Autodesk Inventor part; units mm, degrees
ref_plane "YZ Plane" through (0, 0, 0) normal (1, 0, 0) x (0, 1, 0)
ref_plane "XZ Plane" through (0, 0, 0) normal (0, 1, 0) x (-1, 0, 0)
ref_plane "XY Plane" through (0, 0, 0) normal (0, 0, 1) x (1, 0, 0)
sketch "Эскиз1" plane through (0, 0, 0) normal (0, 0, 1) x (1, 0, 0)
  line L0 (0, 0) -> (35, 0)
  line L1 (35, 0) -> (35, 50)
  line L2 (35, 50) -> (0, 50)
  line L3 (0, 50) -> (0, 0)
  dimension "d0" = 35
  dimension "d1" = 50
extrude "Выдавливание1" add sketch "Эскиз1" along normal blind 1.8
sketch "Эскиз2" plane through (0, 0, 1.8) normal (0, 0, 1) x (1, 0, 0)
  line L0 (0, 0) -> (35, 0)
  line L1 (35, 0) -> (35, 1.8)
  line L2 (35, 1.8) -> (0, 1.8)
  line L3 (0, 1.8) -> (0, 0)
  dimension "d5" = 35
  dimension "d6" = 1.8
extrude "Выдавливание2" add sketch "Эскиз2" along normal blind 48.2
fillet "Сопряжение1" radius 2 2 edges at (17.5, 1.8, 1.8) (17.5, 0, 0)
chamfer "Фаска1" distance 5.175 angle 45 4 edges at (0, 50, 0.9) (0, 0.9, 50) (35, 0.9, 50) (35, 50, 0.9)
sketch "Эскиз3" plane through (0, 0, 1.8) normal (0, 0, 1) x (1, 0, 0)
  line L0 (29.825, 50) -> (5.175, 50)
  line L1 (17.5, 50) -> (17.5, 1.8)
  line L2 (0, 1.8) -> (35, 1.8)
  line L3 (29.825, 50) -> (5.175, 50)
  circle A0 centre (17.5, 39.6875) radius 5
  circle A1 centre (7.9375, 44.6875) radius 2
  circle A2 centre (26.9875, 44.6875) radius 2
  circle A3 centre (5.175, 33.3375) radius 2
  circle A4 centre (29.825, 33.3375) radius 2
  circle A5 centre (7.9375, 20.6375) radius 2
  circle A6 centre (26.9875, 20.6375) radius 2
  point P0 (0, 0)
  dimension "d14" = 10
  dimension "d15" = 4
  dimension "d16" = 4
  dimension "d17" = 4
  dimension "d18" = 4
  dimension "d19" = 4
  dimension "d20" = 4
extrude "Выдавливание3" cut sketch "Эскиз3" against normal blind 48.2
sketch "Эскиз4" plane through (0, 1.8, 3.8) normal (0, 1, 0) x (1, 0, 0)
  line L0 (5.175, -46.2) -> (29.825, -46.2)
  line L1 (5.175, -46.2) -> (29.825, -46.2)
  circle A0 centre (17.5, -35.8875) radius 5
  circle A1 centre (27.0625, -40.8875) radius 2
  circle A2 centre (8.0125, -40.8875) radius 2
  circle A3 centre (29.825, -29.5375) radius 2
  circle A4 centre (5.175, -29.5375) radius 2
  circle A5 centre (27.0625, -16.8375) radius 2
  circle A6 centre (8.0125, -16.8375) radius 2
  line L2 (29.825, -46.2) -> (5.175, -46.2)
  point P0 (0, 3.8)
  point P1 (17.5, -46.2)
  dimension "d23" = 10
  dimension "d24" = 4
  dimension "d25" = 4
  dimension "d26" = 4
  dimension "d27" = 4
  dimension "d28" = 4
  dimension "d29" = 4
extrude "Выдавливание4" cut sketch "Эскиз4" against normal blind 48.2
properties part number "угол для катушки"
Model file for the job. Use its own axes, mm. A direction names the side the tool comes from. Coordinates: 2 decimals unless noted, no trailing zeros. Write each loop counter-clockwise with the first axis right and the second up, starting at its lowest first coordinate (ties: lowest second). Pieces come first, ordered by that corner, then holes. Notation, with made-up numbers: (56, 54) -> (70, 54) arc R4 ccw to (70, 61) -> close; hole circle Ø9 at (44.25, 39.5). An arc over 180 degrees is marked (long way). One line per item, written item: value. Start each with the question number.
1) Which spindle directions (+Z, -Z, +X, -X, +Y, -Y) get a long thin tool onto all of the face, cutting with end or side? Do faces 4 (the face through (17.74, 0.57, 0.6)), 5 (the face through (17, 27, 1.8)). Say none if no direction does.
2) Flat gauge pins, fed straight in: pin 1 Ø4.5 at (x, y) = (26.99, 20.64) entering from -Z; pin 2 Ø8 at (x, y) = (18.5, 30.5) entering from +Z; pin 3 Ø10 at (x, z) = (20.5, 7) entering from +Y; pin 4 Ø4.5 at (x, z) = (5.18, 33.34) entering from +Y. Where does each tip first touch, or does it go through?
3) Slice it at C-C on z = 20. Write the cut outline in (x, y).
4) Slice it at D-D on z = 39. Write the cut outline in (x, y).
5) Pull direction X, two halves, no side cores. Call faces 1 (the face through (2.624, 0.887, 47.449)), 2 (the face through (25.4, 19.42, 0.91)), 3 (the face through (18, 1.8, 27)): +X half, -X half, draft (parallel to the pull), parting line (faces both ways), or undercut.
6) Slice it at B-B on y = 41. Write the cut outline in (x, z), then the cut area to 3 significant figures.
7) Slice it at A-A on x = 17.5. Write the cut outline in (y, z), then the cut area to 3 significant figures.
8) Probe probe 1 along Z at (x, y) = (27, 36.5); probe 2 along Z at (x, y) = (13.5, 2). List the from-to ranges inside material, lowest first.
Answers follow:
1. face 4: -Z, +X, -X, -Y
1. face 5: +Z, +X, -X, +Y
2. pin 1: z = 0
2. pin 2: z = 1.8
2. pin 3: y = 2.93
2. pin 4: y = 1.8
3. outline: (0, 0) -> (6.12, 0) -> (6.12, 1.8) -> (0, 1.8) -> close; (9.91, 0) -> (25.17, 0) -> (25.17, 1.8) -> (9.91, 1.8) -> close; (28.96, 0) -> (35, 0) -> (35, 1.8) -> (28.96, 1.8) -> close
4. outline: (0, 0) -> (12.55, 0) -> (12.55, 1.8) -> (0, 1.8) -> close; (22.45, 0) -> (35, 0) -> (35, 1.8) -> (22.45, 1.8) -> close
5. face 1: -X half
5. face 2: undercut
5. face 3: draft
6. outline: (0, 0) -> (12.68, 0) -> (12.68, 1.8) -> (0, 1.8) -> close; (22.32, 0) -> (35, 0) -> (35, 1.8) -> (22.32, 1.8) -> close
6. area: 45.6 mm2
7. outline: (0, 2) arc R2 ccw to (2, 0) -> (34.69, 0) -> (34.69, 1.8) -> (3.8, 1.8) arc R2 cw to (1.8, 3.8) -> (1.8, 34.69) -> (0, 34.69) -> close; (0, 44.69) -> (1.8, 44.69) -> (1.8, 50) -> (0, 50) -> close; (44.69, 0) -> (50, 0) -> (50, 1.8) -> (44.69, 1.8) -> close
7. area: 141 mm2
8. probe 1: 0 to 1.8
8. probe 2: 0 to 2.93
